Verification items for this drawing (mm, ordinates from the low corner). Round coordinates to 2 decimals unless told otherwise and drop trailing zeros. Order: outer loops, then holes, each group sorted by start corner. A loop starts at its lowest first (then second) coordinate and runs counter-clockwise, first axis right, second up. Notation, with made-up numbers: M 38.25,38 L 57.25,38 A31 ccw 57.25,74 Z; hole C -24.75,77 d6. An arc over 180 degrees is marked long. Return JSON: item names as keys, results as strings. Group by question number.
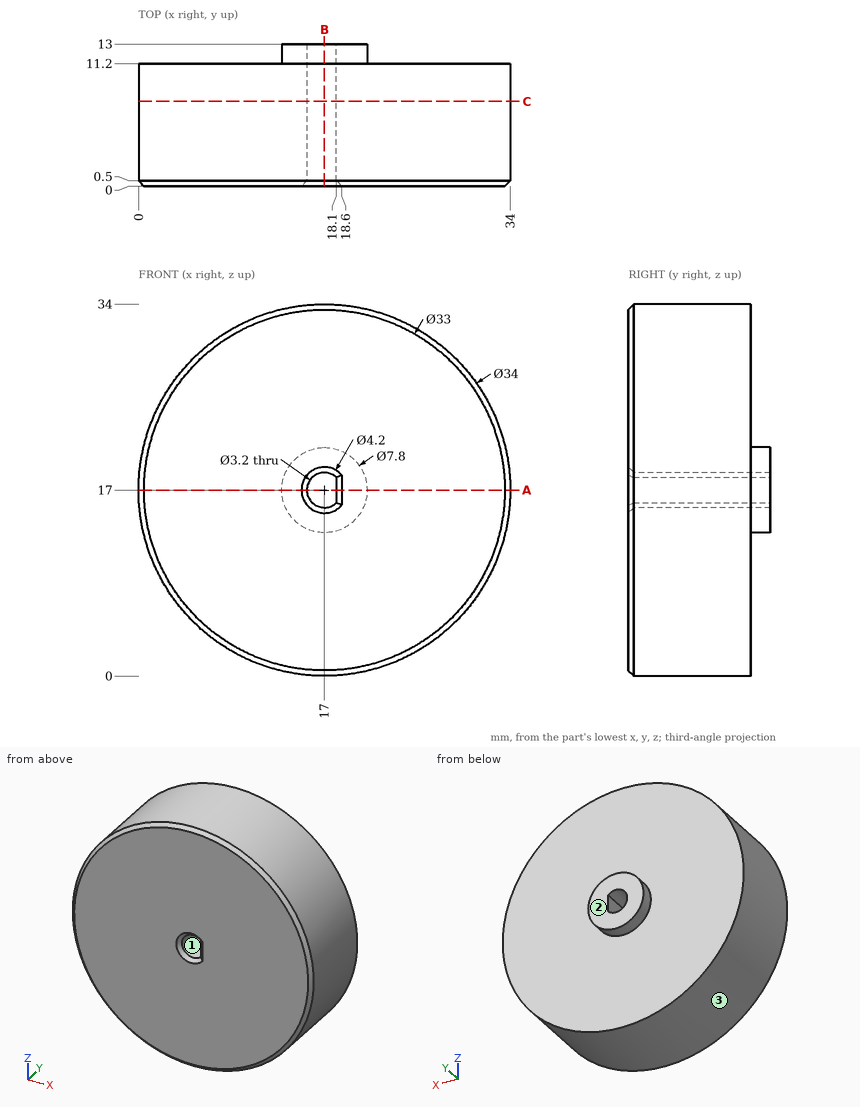
1. Cross-section at A-A (z = 17). Enter the section's corners in (x, y), plus the area to 3 significant figures.
2. Draft check along Z on the marked faces 1, 2 and 3. Enter one of: +Z half, -Z half, draft (parallel to the pull), parting line (faces both ways), or undercut.
3. Thickness scan on line 1 along Y through (x, z) = (27, 14.5); line 2 along Z through (x, y) = (10.5, 2.75); line 3 along X through (y, z) = (9, 12). Record the ranges inside material, lowest first. Write a range as from..to.
4. Cross-section at C-C (y = 7.75). Enter the section's corners in (x, z), plus the area to 3 significant figures.
5. Cross-section at B-B (x = 17). Enter the section's corners in (y, z), plus the area to 3 significant figures.
6. Go/stop test with flat-tipped pins: pin 1 (2 mm diameter, centred on x = 13.5, z = 11.5, fed in from +Y); pin 2 (4 mm diameter, centred on y = 3.5, z = 14, fed in from +X); pin 3 (6 mm diameter, centred on y = 5, z = 30, fed in from +X). Record where each tip stops, or that it passes through.
Computed:
{
 "1": {"outline": "M 0,0.5 L 0.5,0 L 14.9,0 L 15.4,0.5 L 15.4,13 L 13.1,13 L 13.1,11.2 L 0,11.2 Z; M 18.1,0.5 L 18.6,0 L 33.5,0 L 34,0.5 L 34,11.2 L 20.9,11.2 L 20.9,13 L 18.1,13 Z", "area": "359 mm²"},
 "2": {"face 1": "undercut", "face 2": "draft", "face 3": "parting line"},
 "3": {"line 1": "y = 0..11.2", "line 2": "z = 1.29..32.71", "line 3": "x = 0.75..33.25"},
 "4": {"outline": "C 17,17 d34; hole M 18.1,15.84 L 18.1,18.16 A1.6 ccw long Z", "area": "901 mm²"},
 "5": {"outline": "M 0,0.5 L 0.5,0 L 11.2,0 L 11.2,13.1 L 13,13.1 L 13,15.4 L 0.5,15.4 L 0,14.9 Z; M 0,19.1 L 0.5,18.6 L 13,18.6 L 13,20.9 L 11.2,20.9 L 11.2,34 L 0.5,34 L 0,33.5 Z", "area": "353 mm²"},
 "6": {"pin 1": "stops at y = 11.2", "pin 2": "stops at x = 33.97", "pin 3": "stops at x = 30.75"}
}
